Source: CAD feature listing. Evaluate the final solid. Frame: model axes, mm. Face numbers are marked on the shaded views. A direction names the side the tool comes from. Coordinates: 2 decimals unless noted, no trailing zeros. Loops run counter-clockwise (first coordinate to the right, second up) from the corner with the lowest first, then second, coordinate; pieces in that order, holes last. Notation, with made-up numbers: (29, -32) - (68, -32) arc R7 ccw to (68, -28) - close; hole circle Ø10 at (-2, -10.5). An arc over 180 degrees is marked (long way). Write item = value, one per line. Start each with the question number.
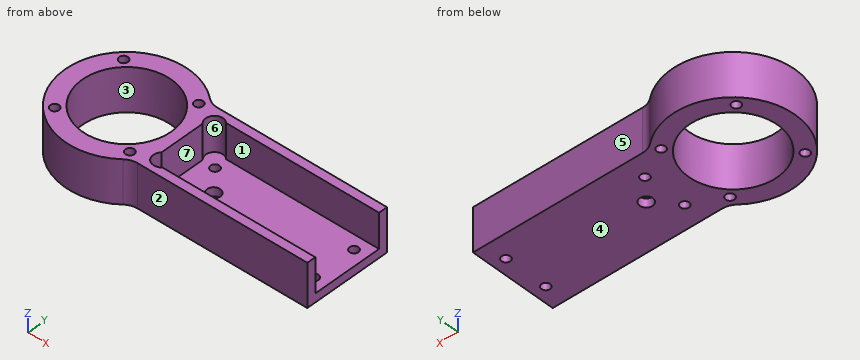
from build123d import *

# Parameters (mm, degrees)
SKETCH1_R               = 32.5
SKETCH1_W               = 120.65
SKETCH1_H               = 50.8
BOSS_EXTRUDE2_DEPTH     = 6.35
BOSS_EXTRUDE3_START     = 6.35
SKETCH1_3_R             = 32.5
BOSS_EXTRUDE3_DEPTH     = 25.4
CUT_EXTRUDE1_DEPTH      = 170.176810751
CUT_EXTRUDE1_DEPTH_BACK = 170.176810751
SKETCH2_R               = 3.175
SKETCH3_R               = 6.35
CUT_EXTRUDE2_DEPTH      = 25.4
SKETCH4_3_R             = 4.7625
CUT_EXTRUDE3_DEPTH      = 6.35
FILLET1_R               = 12.7


with BuildPart() as part:
    # Sketch1 → Boss-Extrude2 (new body)
    # profile 1 of 2: a face of its own
    with BuildSketch(Plane.XY):
        with BuildLine():
            Line((32.171066193, 31.75), (161.036, 31.75))
            Line((161.036, 31.75), (161.036, 25.4))
            Line((161.036, 25.4), (40.386, 25.4))
            Line((40.386, 25.4), (40.386, -25.4))
            Line((40.386, -25.4), (161.036, -25.4))
            Line((161.036, -25.4), (161.036, -31.75))
            Line((161.036, -31.75), (32.171066193, -31.75))
            ThreePointArc((32.171066193, -31.75), (-45.2, 0), (32.171066193, 31.75))
        make_face()
        Circle(SKETCH1_R, mode=Mode.SUBTRACT)
    # profile 2 of 2: a face of its own
    with BuildSketch(Plane.XY):
        with Locations((100.711, 0)):
            Rectangle(SKETCH1_W, SKETCH1_H)
    extrude(amount=BOSS_EXTRUDE2_DEPTH)

    # Sketch1<3> → Boss-Extrude3 (add)
    with BuildSketch(Plane.XY.offset(BOSS_EXTRUDE3_START)):
        with BuildLine():
            Line((32.171066193, 31.75), (161.036, 31.75))
            Line((161.036, 31.75), (161.036, 25.4))
            Line((161.036, 25.4), (40.386, 25.4))
            Line((40.386, 25.4), (40.386, -25.4))
            Line((40.386, -25.4), (161.036, -25.4))
            Line((161.036, -25.4), (161.036, -31.75))
            Line((161.036, -31.75), (32.171066193, -31.75))
            ThreePointArc((32.171066193, -31.75), (-45.2, 0), (32.171066193, 31.75))
        make_face()
        Circle(SKETCH1_3_R, mode=Mode.SUBTRACT)
    extrude(amount=BOSS_EXTRUDE3_DEPTH)

    # Sketch2 → Cut-Extrude1 (cut, two sides: drawn at the far end of the back side and taken through both)
    with BuildSketch(Plane.XY.offset(6.35).offset(-CUT_EXTRUDE1_DEPTH_BACK)):
        with Locations((49.911, 15.875)):
            Circle(SKETCH2_R)
        with Locations((151.511, 15.875)):
            Circle(SKETCH2_R)
        with Locations((151.511, -15.875)):
            Circle(SKETCH2_R)
        with Locations((49.911, -15.875)):
            Circle(SKETCH2_R)
        with Locations((27.471098449, 27.471098449)):
            Circle(SKETCH2_R)
        with Locations((27.471098449, -27.471098449)):
            Circle(SKETCH2_R)
        with Locations((-27.471098449, -27.471098449)):
            Circle(SKETCH2_R)
        with Locations((-27.471098449, 27.471098449)):
            Circle(SKETCH2_R)
    extrude(amount=CUT_EXTRUDE1_DEPTH + CUT_EXTRUDE1_DEPTH_BACK, mode=Mode.SUBTRACT)

    # Sketch3 → Cut-Extrude2 (cut)
    with BuildSketch(Plane.XY.offset(31.75)):
        with Locations((44.876128061, 20.909871939)):
            Circle(SKETCH3_R)
        with Locations((44.876128061, -20.909871939)):
            Circle(SKETCH3_R)
    extrude(amount=-CUT_EXTRUDE2_DEPTH, mode=Mode.SUBTRACT)

    # Sketch4<3> → Cut-Extrude3 (cut)
    with BuildSketch(Plane(origin=(0, 0, 0), x_dir=(-1, 0, 0), z_dir=(0, 0, -1))):
        with Locations((-63.5, 0)):
            Circle(SKETCH4_3_R)
    extrude(amount=-CUT_EXTRUDE3_DEPTH, mode=Mode.SUBTRACT)

    # Fillet1
    fillet1_edges = [part.edges().sort_by_distance(p)[0] for p in [
        (32.171066193, -31.75, 15.875),
        (32.171066193, 31.75, 15.875),
    ]]
    fillet(fillet1_edges, radius=FILLET1_R)


solid = part.part
Item 1: Cut plane B-B (y = 0). Return the cut outline in (x, z), then the cut area to 3 significant figures.
Item 2: First-contact query: pin 1 (3 mm diameter, centred on y = -21.5, z = 22, fed in from +X); pin 2 (2 mm diameter, centred on x = 54, y = -6, fed in from +Z); pin 3 (12.5 mm diameter, centred on x = 79, z = 19.5, fed in from +Y). Flat tips, straight axial feed; report the tip coordinate or a pass-through.
Item 3: Cut plane C-C (y = 21). Return the cut outline in (x, z), then the cut area to 3 significant figures.
Item 4: Cut plane A-A (x = 63.5). Return the cut outline in (y, z), then the cut area to 3 significant figures.
Item 5: Draft query along Y for the marked faces 4, 5, 6 and 7. Return one class per face: released by +Y, released by -Y, zero draft, split by the parting line, or undercut.
Item 6: Cut plane D-D (z = 3.5). State how many separate pieces and enclosed holes the cut face has, then the cut area to 3 significant figures.
Item 7: Material intervals for L1, parallel to Y at x = 100.5, z = 26.5; L2, parallel to X at y = -0.5, z = 19; L3, parallel to X at y = 25.5, z = 30, sorted ascending. Write a range as [from, to].
Item 8: Reachability of the marked faces 1, 2 and 3 from +Z, -Z, +X, -X, +Y, -Y: full face, straight path, thin tool, end or side. Return the list, or none.
Responses:
q1.outline = (-45.2, 0) - (-32.5, 0) - (-32.5, 31.75) - (-45.2, 31.75) - close; (32.5, 0) - (58.74, 0) - (58.74, 6.35) - (40.39, 6.35) - (40.39, 31.75) - (32.5, 31.75) - close; (68.26, 0) - (161.04, 0) - (161.04, 6.35) - (68.26, 6.35) - close
q1.area = 1,360 mm2
q2.pin_1 = 38.88
q2.pin_2 = 6.35
q2.pin_3 = 31.75
q3.outline = (-40.03, 0) - (-24.8, 0) - (-24.8, 31.75) - (-40.03, 31.75) - close; (24.8, 0) - (161.04, 0) - (161.04, 6.35) - (38.53, 6.35) - (38.53, 31.75) - (24.8, 31.75) - close
q3.area = 1,700 mm2
q4.outline = (-31.75, 0) - (-4.76, 0) - (-4.76, 6.35) - (-25.4, 6.35) - (-25.4, 31.75) - (-31.75, 31.75) - close; (4.76, 0) - (31.75, 0) - (31.75, 31.75) - (25.4, 31.75) - (25.4, 6.35) - (4.76, 6.35) - close
q4.area = 665 mm2
q5.face_4 = zero draft
q5.face_5 = released by +Y
q5.face_6 = undercut
q5.face_7 = undercut
q6.separate_pieces = 1
q6.enclosed_holes = 10
q6.area = 10,400 mm2
q7.L1 = [-31.75, -25.4], [25.4, 31.75]
q7.L2 = [-45.2, -32.5], [32.5, 40.39]
q7.L3 = [-37.32, -29.96], [-24.98, -20.15], [20.15, 24.98], [29.96, 40.49], [49.26, 161.04]
q8.face_1 = +Z, +X
q8.face_2 = +Z, -Z, +X, -Y
q8.face_3 = +Z, -Z
